Study the drawing (mm; zero at the part's minimum x, y, z) and answer. A direction names the side the tool comes from. Round coordinates to 2 decimals unless told otherwise and drop trailing zeros. Order: outer loops, then holes, each group sorted by start corner. A loop starts at its lowest first (then second) coordinate and runs counter-clockwise, first axis right, second up. Notation, with made-up numbers: M 79.25,46 L 111.25,46 A8 ccw 111.25,59 Z; hole C -34.75,75 d7. An arc over 180 degrees is marked long. Put each result on its own line as item: value. Start each with the question number.
1. The part is cut by section A-A (x = 15). Give the vertices of the cut face in (y, z).
2. The part is cut by section C-C (y = 15). Count the separate pieces of the cut face and the enclosed holes in it, then the cut area to 3 significant figures.
3. Consider line 1 (Y direction, x = 15, z = 24.5); line 2 (Z direction, x = 17, y = 28); line 3 (X direction, y = 15.5, z = 9). Determine where each line is inside the solid, lowest interval first.
4. The part is cut by section B-B (z = 21). Give the vertices of the cut face in (x, y).
5. Each of these flat-tipped pins is pushed along its axis until it touches: pin 1 Ø4 at (x, z) = (24.5, 28) entering from +Y; pin 2 Ø5 at (x, z) = (19, 32) entering from +Y (1 decimal); pin 3 Ø5 at (y, z) = (9.5, 29) entering from -X. Where does it stop, or does it pass through?
6. The mould has two halves that part along Y. Classify the marked faces 3, 4 and 5: +Y half, -Y half, draft (parallel to the pull), parting line (faces both ways), or undercut.
7. Which of the six approach directions +Z, -Z, +X, -X, +Y, -Y give full straight-line access (tool end or side, diameter ignored) to the marked faces 1 and 2?
8. The part is cut by section D-D (x = 21.5). Give the vertices of the cut face in (y, z).
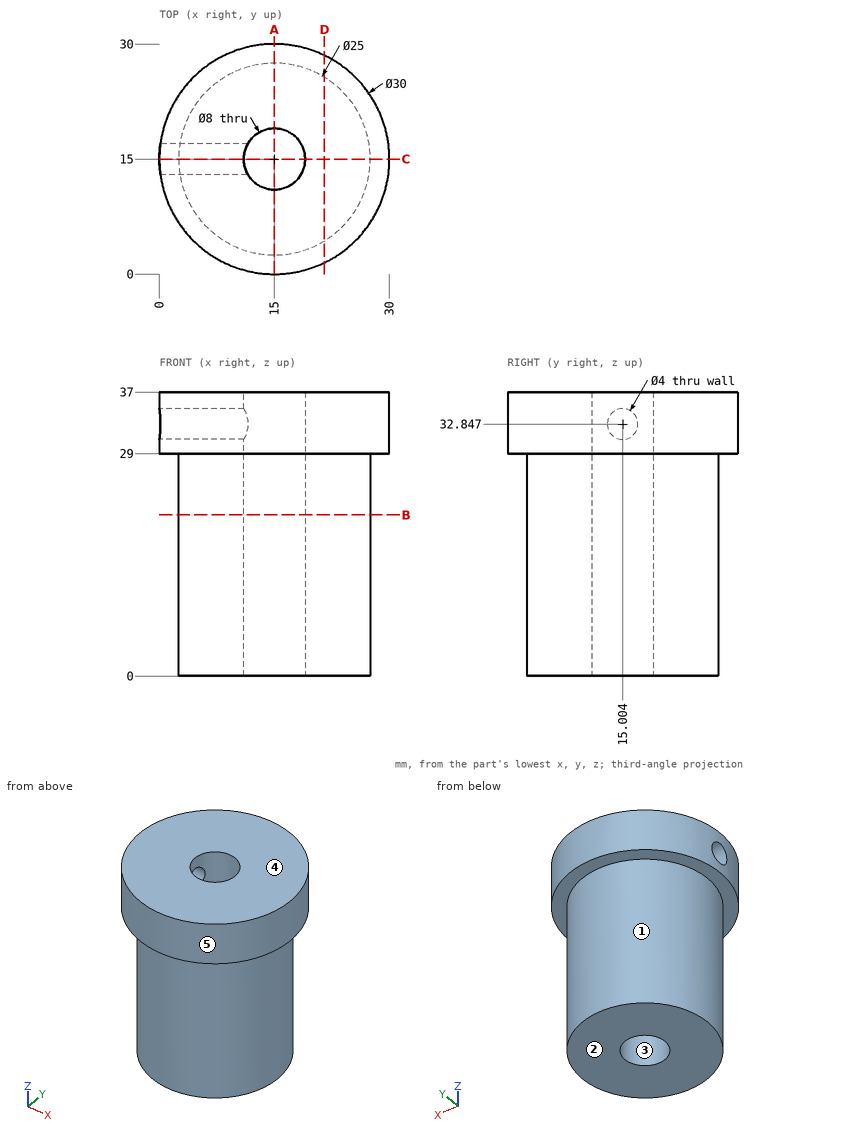
Resolved:
1. outline: M 0,29 L 2.5,29 L 2.5,0 L 11,0 L 11,37 L 0,37 Z; M 19,0 L 27.5,0 L 27.5,29 L 30,29 L 30,37 L 19,37 Z
2. separate pieces: 3
2. enclosed holes: 0
2. area: 625 mm2
3. line 1: 2.5 to 11, 19 to 27.5
3. line 2: 29 to 37
3. line 3: 2.51 to 11.03, 18.97 to 27.49
4. outline: C 15,15 d25; hole C 15,15 d8
5. pin 1: y = 27.83
5. pin 2: y = 29.9
5. pin 3: x = 0.3
6. face 3: undercut
6. face 4: draft
6. face 5: parting line
7. face 1: -Z
7. face 2: -Z, +X, -X, +Y, -Y
8. outline: M 1.48,29 L 4.32,29 L 4.32,0 L 25.68,0 L 25.68,29 L 28.52,29 L 28.52,37 L 1.48,37 Z
